Build history of the part. All positions in model axes, mm. A direction names the side the tool comes from. Round coordinates to 2 decimals unless told otherwise and drop trailing zeros. Write each loop counter-clockwise with the first axis right and the second up, starting at its lowest first coordinate (ties: lowest second). Pieces come first, ordered by that corner, then holes. Notation, with made-up numbers: (32, -14) - (81, -14) arc R15 ccw to (81, 0) - close; hole circle Ø6 at (65.5, 6.25). An arc over 180 degrees is marked (long way). Answer as a JSON object with one key per item and string values. Group by question number.
Item 1: Two-plate mould, pull along X, no slides. Class faces 1 (the cylindrical face through (-292.3, -66.23, 3.13)), 2 (the cylindrical face through (-435.94, -34.01, 3.13)), 3 (the cylindrical face through (-260.23, 297.69, 3.13)): +X half, -X half, draft (parallel to the pull), parting line (faces both ways), or undercut.
Item 2: Which spindle directions (+Z, -Z, +X, -X, +Y, -Y) get a long thin tool onto all of the face, cutting with end or side? Do faces 4 (the flat face through (-249.693, 45.469, 3.131)), 5 (the flat face through (-189, 134, 6.35)). Say none if no direction does.
Item 3: Slice it at D-D, the plane y = 186. List the corners of the cut face in (x, z).
Item 4: Slice it at B-B, the plane z = 5. Give the number of separate pieces and of enclosed holes in the cut face, then the cut area to 3 significant figures.
Item 5: Slice it at A-A, the plane y = 88. List the corners of the cut face in (x, z), then the cut area to 3 significant figures.
Item 6: Slice it at C-C, the plane y = 276. List the corners of the cut face in (x, z).
Item 7: Flat gauge pins, fed straight in: pin 1 (3 mm diameter, centred on x = -3, z = 4.5, fed in from -Y) (3 decimals); pin 2 (23 mm diameter, centred on x = -134.04, y = 139.7, fed in from +Z); pin 3 (2 mm diameter, centred on y = 251, z = 2, fed in from -X); pin 4 (3 mm diameter, centred on y = -44, z = 4, fed in from +X). Where does each tip first touch, or does it go through?
Item 8: Probe line 1 (X direction, y = 137, z = 2.25); line 2 (X direction, y = 266, z = 4.25); line 3 (X direction, y = -18.5, z = 0.75). List the from-to ranges inside material, lowest first. Write a range as from..to.
from build123d import *

# Parameters (mm, degrees)
MODEL_R             = 2.4892
MODEL_R_2           = 14.351
MODEL_R_3           = 19.05
BOSS_EXTRUDE1_DEPTH = 6.35


with BuildPart() as part:
    # Model → Boss-Extrude1 (new body)
    with BuildSketch(Plane.XY):
        with BuildLine():
            Line((-441.789312, -6.889165677), (-441.789312, -25.038634323))
            ThreePointArc((-441.789312, -25.038634323), (-435.829532347, -34.118973304), (-426.62152736, -39.879543908))
            Line((-426.62152736, -39.879543908), (-346.203265936, -68.649155922))
            ThreePointArc((-346.203265936, -68.649155922), (-342.794136372, -69.547563331), (-339.28161131, -69.85))
            Line((-339.28161131, -69.85), (-301.18161131, -69.85))
            ThreePointArc((-301.18161131, -69.85), (-292.201355189, -66.130256121), (-288.48161131, -57.15))
            Line((-288.48161131, -57.15), (-288.48161131, -15.263054603))
            ThreePointArc((-288.48161131, -15.263054603), (-287.916123528, -11.515573687), (-286.270018677, -8.101817916))
            Line((-286.270018677, -8.101817916), (-212.077490922, 100.561181044))
            ThreePointArc((-212.077490922, 100.561181044), (-207.671459082, 104.548698007), (-201.933730241, 106.095267065))
            Line((-201.933730241, 106.095267065), (-145.278114328, 107.633327242))
            ThreePointArc((-145.278114328, 107.633327242), (-141.931465661, 107.278101134), (-138.795626118, 106.056318319))
            Line((-138.795626118, 106.056318319), (-87.594102076, 77.790625657))
            ThreePointArc((-87.594102076, 77.790625657), (-82.794837325, 73.127519562), (-81.0319436, 66.672311872))
            Line((-81.0319436, 66.672311872), (-81.0319436, -9.525))
            ThreePointArc((-81.0319436, -9.525), (-77.312199721, -18.505256121), (-68.3319436, -22.225))
            Line((-68.3319436, -22.225), (58.6680564, -22.225))
            ThreePointArc((58.6680564, -22.225), (67.648312521, -18.505256121), (71.3680564, -9.525))
            Line((71.3680564, -9.525), (71.3680564, 43.162005366))
            ThreePointArc((71.3680564, 43.162005366), (70.286480643, 48.290574182), (67.225974809, 52.545609817))
            Line((67.225974809, 52.545609817), (-231.724912696, 325.191085975))
            ThreePointArc((-231.724912696, 325.191085975), (-253.238197861, 331.440320626), (-271.33067791, 318.229092902))
            Line((-271.33067791, 318.229092902), (-440.555640395, -4.158684171))
            ThreePointArc((-440.555640395, -4.158684171), (-441.212773023, -5.505718227), (-441.789312, -6.889165677))
        make_face()
        with Locations((58.6680564, 42.418)):
            Circle(MODEL_R, mode=Mode.SUBTRACT)
        with Locations((-248.840749515, 306.423877073)):
            Circle(MODEL_R_2, mode=Mode.SUBTRACT)
        with Locations((-232.729624751, 269.086142594)):
            Circle(MODEL_R_2, mode=Mode.SUBTRACT)
        with Locations((-134.044120223, 165.1)):
            Circle(MODEL_R, mode=Mode.SUBTRACT)
        with Locations((-68.3319436, 42.418)):
            Circle(MODEL_R, mode=Mode.SUBTRACT)
        with Locations((-134.044120223, 114.3)):
            Circle(MODEL_R, mode=Mode.SUBTRACT)
        with Locations((58.6680564, -14.732)):
            Circle(MODEL_R, mode=Mode.SUBTRACT)
        with Locations((-339.28161131, -49.3014)):
            Circle(MODEL_R_2, mode=Mode.SUBTRACT)
        with Locations((-418.065712, -15.9639)):
            Circle(MODEL_R_2, mode=Mode.SUBTRACT)
        with Locations((-222.079312, 130.957722259)):
            Circle(MODEL_R_2, mode=Mode.SUBTRACT)
        with Locations((-134.044120223, 139.7)):
            Circle(MODEL_R_3, mode=Mode.SUBTRACT)
        with Locations((-68.3319436, -14.732)):
            Circle(MODEL_R, mode=Mode.SUBTRACT)
    extrude(amount=BOSS_EXTRUDE1_DEPTH)


solid = part.part
Geometry says:
{
 "1": {"face 1": "+X half", "face 2": "-X half", "face 3": "undercut"},
 "2": {"face 4": "+Z, -Z, -Y", "face 5": "+Z, +X, -X, +Y, -Y"},
 "3": {"outline": "(-340.74, 0) - (-79.1, 0) - (-79.1, 6.35) - (-340.74, 6.35) - close"},
 "4": {"separate pieces": "1", "enclosed holes": "12", "area": "87,600 mm^2"},
 "5": {"outline": "(-392.18, 0) - (-220.65, 0) - (-220.65, 6.35) - (-392.18, 6.35) - close; (-106.09, 0) - (28.35, 0) - (28.35, 6.35) - (-106.09, 6.35) - close", "area": "1,940 mm^2"},
 "6": {"outline": "(-293.5, 0) - (-245.31, 0) - (-245.31, 6.35) - (-293.5, 6.35) - close; (-220.15, 0) - (-177.79, 0) - (-177.79, 6.35) - (-220.15, 6.35) - close"},
 "7": {"pin 1": "stops at y = -22.225", "pin 2": "passes through", "pin 3": "stops at x = -307.14", "pin 4": "stops at x = -288.48"},
 "8": {"line 1": "x = -366.46..-235.1, -209.06..-152.9, -115.19..-25.38", "line 2": "x = -298.75..-246.74, -218.71..-166.82", "line 3": "x = -441.79..-432.19, -403.94..-288.48, -77.32..67.65"}
}
